from build123d import *

# Parameters (mm, degrees)
SKETCH1_W                = 20
SKETCH1_H                = 20
BOSS_EXTRUDE1_DEPTH      = 1
BOSS_EXTRUDE5_DEPTH      = 20
BOSS_EXTRUDE6_DEPTH      = 5
BOSS_EXTRUDE6_DEPTH_BACK = 5
SKETCH5_W                = 1.5
SKETCH5_H                = 20
CUT_EXTRUDE1_DEPTH       = 5
BOSS_EXTRUDE7_DEPTH      = 1.5


with BuildPart() as part:
    # Sketch1 → Boss-Extrude1 (new body)
    with BuildSketch(Plane(origin=(0, 0, 0), x_dir=(1, 0, 0), z_dir=(0, 1, 0))):
        Rectangle(SKETCH1_W, SKETCH1_H)
    extrude(amount=BOSS_EXTRUDE1_DEPTH)

    # Sketch4 → Boss-Extrude5 (add)
    with BuildSketch(Plane(origin=(10, 0, 0), x_dir=(0, 0, -1), z_dir=(1, 0, 0))):
        Polygon((-2, 0), (-2, -2), (-4.5, -2), (-4.5, -3.436102186), (4.5, -3.436102186), (4.5, -2), (2, -2), (2, 0), align=None)
    extrude(amount=-BOSS_EXTRUDE5_DEPTH)



with BuildPart() as body_2:
    # Sketch5 → Boss-Extrude6 (new, two sides: drawn at the far end of the back side and taken through both)
    with BuildSketch(Plane.ZY.offset(10).offset(-BOSS_EXTRUDE6_DEPTH_BACK)):
        with Locations((-1.65, 11)):
            Rectangle(SKETCH5_W, SKETCH5_H)
    extrude(amount=BOSS_EXTRUDE6_DEPTH + BOSS_EXTRUDE6_DEPTH_BACK)

    # Sketch6 → Cut-Extrude1 (cut)
    with BuildSketch(Plane.XY.offset(-0.9)):
        Polygon((-5, 1), (-10, 21), (-5, 21), align=None)
    extrude(amount=-CUT_EXTRUDE1_DEPTH, mode=Mode.SUBTRACT)


with BuildPart() as part_1:
    add(part.part)

    add(body_2.part)  # Boss-Extrude7 merges body 2
    # Sketch5_3 → Boss-Extrude7 (add)
    with BuildSketch(Plane.ZY.offset(10)):
        Polygon((-10, 1), (-2.4, 1), (-2.4, 21), align=None)
        Polygon((-0.9, 0), (-0.9, 1), (-2.4, 1), (-10, 1), (-10, 0), (-2, 0), align=None)
    extrude(amount=BOSS_EXTRUDE7_DEPTH)

    # Mirror5: part across plane


with BuildPart() as part_2:
    add(part_1.part)
    add(part_1.part.mirror(Plane.XY))


solid = part_2.part
The listing builds one solid part. Answer for the finished solid, in the listing's coordinates (mm). A direction names the side the tool comes from. Give positions to 0.01 mm unless a question says otherwise; leave off trailing zeros. Write each loop counter-clockwise with the first axis right and the second up, starting at its lowest first coordinate (ties: lowest second). Pieces come first, ordered by that corner, then holes.
1) For a pull along Y with two mould halves and no side action, classify faces 1 (the face through (-7.465, 10.86, -1.64)), 2 (the face through (-13, 1, 2)), 3 (the face through (-10, 7, -5)), 4 (the face through (-1, 0, 6)) as pulls with the +Y half, pulls with the -Y half, needs draft (parallel to the pull), parting line crosses it, or undercut.
2) Given P1, Ø4, axis at y = 13, z = 8, coming from the +X side; P2, Ø5.5, axis at x = -8.5, y = 8, coming from the -Z side; P3, Ø1.6, axis at x = -13.5, z = -1.5, coming from the -Y side; P4, Ø4, axis at y = 12.5, z = -7.5, coming from the +X side, each flat-ended and moving along its own axis, determine where each tip first touches the part or whether it passes through.
3) Section B-B (x = -13) is taken. Write down the section's boundary in (y, z), and give its area (3 significant figures).
4) A tool of negligible diameter and unlimited length cuts with its end or side. For faces 5 (the face through (-13, 11, 2.4)), 6 (the face through (0, -3, 4.5)), 7 (the face through (-10, 7, 5)), 8 (the face through (-13, 1, -2)), from which of +Z, -Z, +X, -X, +Y, -Y can it reach the whole face along a straight path? Write none if from no direction.
5) Find the intervals of material crossed by L1, parallel to Z at x = -9, y = 5.75; L2, parallel to Y at x = 0, z = -5.75; L3, parallel to Y at x = 0.5, z = -3.25, in increasing order.
6) Section A-A (y = 9) is taken. Write down the section's boundary in (x, z).
7) Section D-D (z = 5.25) is taken. Write down the section's boundary in (x, y), and give its area (4 significant figures).
8) Section C-C (x = 0.5) is taken. Write down the section's boundary in (y, z), and give its area (3 significant figures).
Response:
1. face 1: pulls with the +Y half
1. face 2: pulls with the -Y half
1. face 3: needs draft
1. face 4: undercut
2. P1: passes through
2. P2: stops at z = -8.22
2. P3: stops at y = 1
2. P4: stops at x = -10
3. outline: (1, -2.4) - (21, -2.4) - (21, -0.9) - (1, -0.9) - close; (1, 0.9) - (21, 0.9) - (21, 2.4) - (1, 2.4) - close
3. area: 60.0 mm2
4. face 5: +Z, -X, +Y, -Y
4. face 6: +Z, +X, -X, -Y
4. face 7: +Z, +X, +Y
4. face 8: +Z, -Z, -X, -Y
5. L1: z = -2.4 to -0.9, 0.9 to 2.4
5. L2: y = 0 to 1
5. L3: y = -3.44 to -2, 0 to 1
6. outline: (-15, -2.4) - (-11.5, -2.4) - (-11.5, -6.96) - (-10, -6.96) - (-10, -2.4) - (-7, -2.4) - (-7, -0.9) - (-15, -0.9) - close; (-15, 0.9) - (-7, 0.9) - (-7, 2.4) - (-10, 2.4) - (-10, 6.96) - (-11.5, 6.96) - (-11.5, 2.4) - (-15, 2.4) - close
7. outline: (-11.5, 0) - (10, 0) - (10, 1) - (-10, 1) - (-10, 13.5) - (-11.5, 13.5) - close
7. area: 40.25 mm2
8. outline: (-3.44, -4.5) - (-2, -4.5) - (-2, -2) - (0, -2) - (0, -10) - (1, -10) - (1, 10) - (0, 10) - (0, 2) - (-2, 2) - (-2, 4.5) - (-3.44, 4.5) - close
8. area: 40.9 mm2
